Check sheet for the modelled part. Datum: model origin and axes. Units: mm. Give positions to 0.01 mm unless a question says otherwise; leave off trailing zeros. Write each loop counter-clockwise with the first axis right and the second up, starting at its lowest first coordinate (ties: lowest second). Pieces come first, ordered by that corner, then holes. Notation, with made-up numbers: (34.5, 74) -> (62.5, 74) arc R12 cw to (62.5, 84) -> close; hole circle Ø9 at (51, 22). An arc over 180 degrees is marked (long way). Use a Markdown table: item, result. Add a question column.
1. Cross-section at B-B (y = -20). Enter the section's corners in (x, z).
2. Cross-section at A-A (z = -47.5). Enter the section's corners in (x, y) (3 decimals), then the cut area to 3 significant figures.
3. Scan lines: probe 1 along Z at (x, y) = (13, 11.5); probe 2 along Y at (x, z) = (17.75, -19.5) (3 decimals); probe 3 along Z at (x, y) = (12.75, -27). Record each from-to range of solid material in increasing order. Write a range as [from, to].
4. Cross-section at C-C (x = 8.75). Enter the section's corners in (y, z), then the cut area to 3 significant figures.
5. Gauge pin test, flat ends, axial feed: P1, Ø1.5, axis at x = 4.5, z = 89.5, coming from the +Y side; P2, Ø3, axis at x = 15, z = -105.5, coming from the -Y side; P3, Ø1, axis at x = 16, z = 127, coming from the -Y side. Record the tip position at first contact, or that the pin passes through.
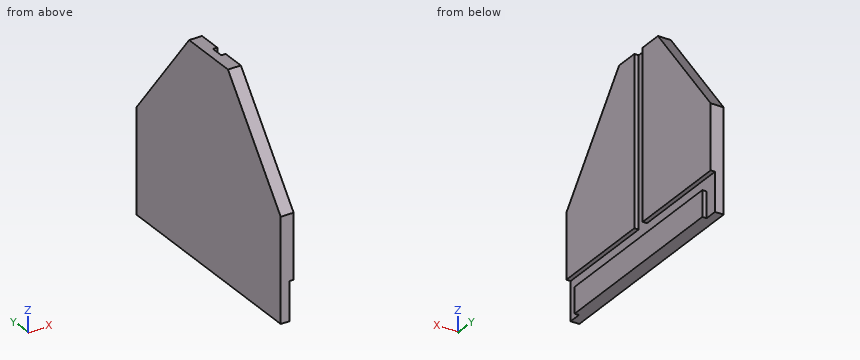
from build123d import *

# Parameters (mm, degrees)
F1_DEPTH = 19.05
F2_W     = 6.35
F2_H     = 19.05
F3_DEPTH = 330.2
F4_W     = 6.35
F4_H     = 19.05
F5_DEPTH = 38.1
F6_W     = 6.35
F6_H     = 19.05
F7_DEPTH = 247.65


# Not quite as in the source:
# - a feature names something its author has since deleted; it is built from what else it names


with BuildPart() as f1:
    # F0 (on Right) → F1 (new body)
    with BuildSketch(Plane.YZ):
        Polygon((-120.65, 27.2672971964), (-120.65, -125.1327028036), (209.55, -125.1327028036), (209.55, 27.2672971964), (88.9, 179.6672971964), (0, 179.6672971964), align=None)
    extrude(amount=F1_DEPTH)

    # F2 (on face) → F3 (cut)
    with BuildSketch(Plane.XZ.offset(120.65)):
        with Locations((15.875, -77.5077028036)):
            Rectangle(F2_W, F2_H)
    extrude(amount=-F3_DEPTH, mode=Mode.SUBTRACT)

    # F4 (on face) → F5 (cut)
    with BuildSketch(Plane(origin=(0, 0, -125.1327028036), x_dir=(1, 0, 0), z_dir=(0, 0, -1))):
        with Locations((15.875, 111.125)):
            Rectangle(F4_W, F4_H)
        with Locations((15.875, -200.025)):
            Rectangle(F4_W, F4_H)
    extrude(amount=-F5_DEPTH, mode=Mode.SUBTRACT)

    # F6 (on face) → F7 (cut)
    with BuildSketch(Plane.XY.offset(179.6672971964)):
        with Locations((15.875, 44.45)):
            Rectangle(F6_W, F6_H)
    extrude(amount=-F7_DEPTH, mode=Mode.SUBTRACT)


solid = f1.part
Worked answers:
| question | item | result |
|---|---|---|
| 1 | outline | (0, -125.13) -> (19.05, -125.13) -> (19.05, -87.03) -> (12.7, -87.03) -> (12.7, -67.98) -> (19.05, -67.98) -> (19.05, 154.4) -> (0, 154.4) -> close |
| 2 | outline | (0, -120.65) -> (19.05, -120.65) -> (19.05, 34.925) -> (12.7, 34.925) -> (12.7, 53.975) -> (19.05, 53.975) -> (19.05, 209.55) -> (0, 209.55) -> close |
| 2 | area | 6,170 mm² |
| 3 | probe 1 | z = [-125.13, -87.03], [-67.98, 179.67] |
| 3 | probe 2 | y = [-120.65, 34.925], [53.975, 209.55] |
| 3 | probe 3 | z = [-125.13, -87.03], [-67.98, 145.56] |
| 4 | outline | (-120.65, -125.13) -> (209.55, -125.13) -> (209.55, 27.27) -> (88.9, 179.67) -> (0, 179.67) -> (-120.65, 27.27) -> close |
| 4 | area | 82,300 mm² |
| 5 | P1 | stops at y = 160.88 |
| 5 | P2 | stops at y = -101.6 |
| 5 | P3 | stops at y = -42.09 |
